Check sheet for the drawn part. Datum: minimum x, y, z corner. Units: mm. A direction names the side the tool comes from. Round coordinates to 2 decimals unless told otherwise and drop trailing zeros. Write each loop counter-clockwise with the first axis right and the second up, starting at its lowest first coordinate (ties: lowest second). Pieces come first, ordered by that corner, then holes. Notation, with made-up numbers: (14.25, -39.5) - (56.25, -39.5) arc R19 ccw to (56.25, -12.5) - close; hole circle Ø9 at (23, -24). An arc over 180 degrees is marked (long way). Answer as a JSON object with one key per item and string values. Group by question number.
1) Go/stop test with flat-tipped pins: pin 1 Ø2 at (y, z) = (5.5, 29) entering from -X; pin 2 Ø6 at (x, y) = (14.5, 4.5) entering from +Z. Record where each tip stops, or that it passes through.
2) Thickness scan on line 1 (Z direction, x = 11, y = 1.75); line 2 (Z direction, x = 4, y = 11). Record the ranges inside material, lowest first.
3) Section check C-C (x = 34). Enter the section's corners in (y, z).
4) Section check D-D (z = 4.5). Enter the section's corners in (x, y), then the cut area to 3 significant figures.
5) Set-up check for the marked faces 1, 2 and 3: record each of +Z, -Z, +X, -X, +Y, -Y from which the full face is reachable in a straight line by a thin tool's end or side.
6) Section check A-A (z = 28). Enter the section's corners in (x, y).
7) Mould release check, pull along Z, two halves, no side actions. Record for the marked faces 4, 5 and 6: +Z half, -Z half, draft (parallel to the pull), parting line (faces both ways), or undercut.
8) Section check B-B (y = 7). Enter the section's corners in (x, z), then the cut area to 3 significant figures.
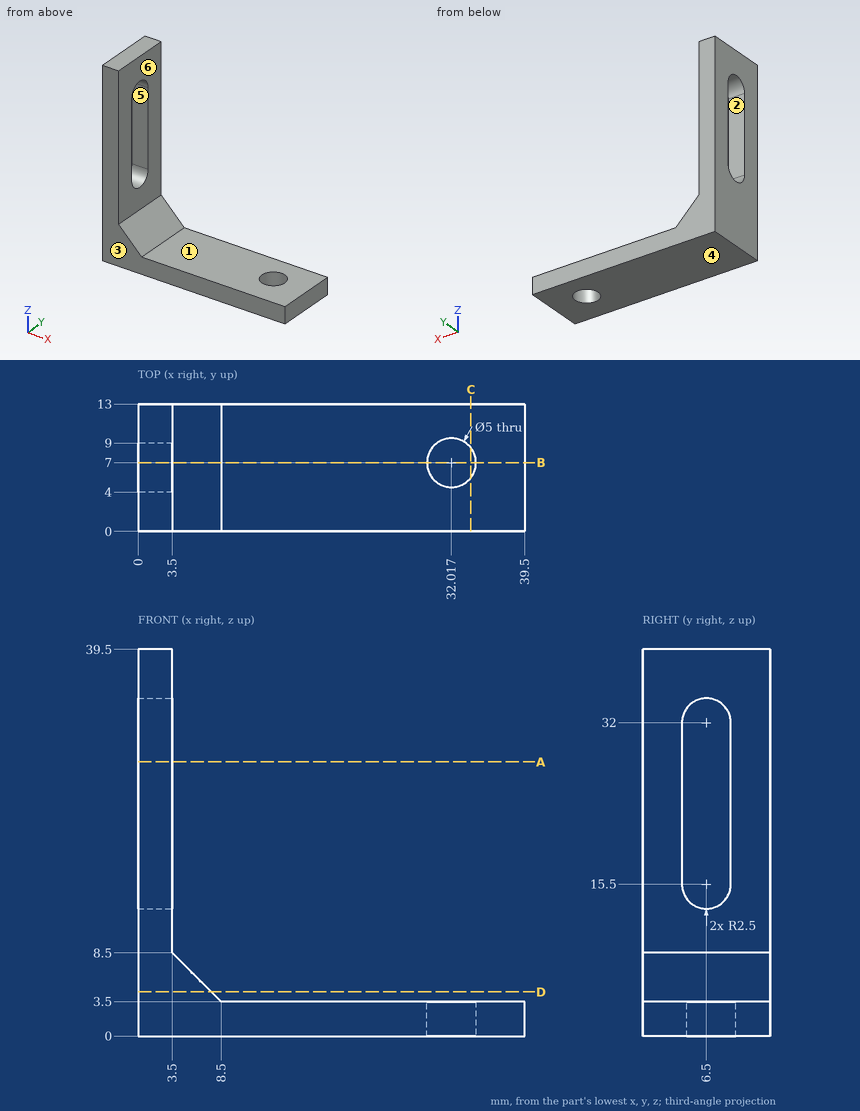
Returned:
{
 "1": {"pin 1": "through", "pin 2": "z = 3.5"},
 "2": {"line 1": "0 to 3.5", "line 2": "0 to 8"},
 "3": {"outline": "(0, 0) - (5.48, 0) - (5.48, 3.5) - (0, 3.5) - close; (8.52, 0) - (13, 0) - (13, 3.5) - (8.52, 3.5) - close"},
 "4": {"outline": "(0, 0) - (7.5, 0) - (7.5, 13) - (0, 13) - close", "area": "97.5 mm2"},
 "5": {"face 1": "+Z, +X, +Y, -Y", "face 2": "+X, -X", "face 3": "+Z, -Z, +X, -X, -Y"},
 "6": {"outline": "(0, 0) - (3.5, 0) - (3.5, 4) - (0, 4) - close; (0, 9) - (3.5, 9) - (3.5, 13) - (0, 13) - close"},
 "7": {"face 4": "-Z half", "face 5": "undercut", "face 6": "draft"},
 "8": {"outline": "(0, 0) - (29.52, 0) - (29.52, 3.5) - (8.5, 3.5) - (3.5, 8.5) - (3.5, 13.05) - (0, 13.05) - close; (0, 34.45) - (3.5, 34.45) - (3.5, 39.5) - (0, 39.5) - close; (34.52, 0) - (39.5, 0) - (39.5, 3.5) - (34.52, 3.5) - close", "area": "184 mm2"}
}
